from build123d import *

# Parameters (mm, degrees)
SKETCH_R     = 2
PAD_DEPTH    = 3
SKETCH001_W  = 5
SKETCH001_H  = 80
PAD001_DEPTH = 11.7
SKETCH002_R  = 1.75
SKETCH002_W  = 45
SKETCH002_H  = 10
POCKET_DEPTH = 15
SKETCH003_W  = 5
SKETCH003_H  = 80
PAD002_DEPTH = 2
FILLET_R     = 8


with BuildPart() as part:
    # Sketch → Pad (new body)
    with BuildSketch(Plane.XY):
        with BuildLine():
            Line((-14.5, 57.5), (14.5, 57.5))
            ThreePointArc((17.5, 54.5), (16.62132, 56.62132), (14.5, 57.5))
            Line((17.5, 54.5), (17.5, 45.5))
            ThreePointArc((14.5, 42.5), (16.62132, 43.37868), (17.5, 45.5))
            Line((14.5, 42.5), (5, 42.5))
            Line((5, 42.5), (5, -42.5))
            Line((5, -42.5), (14.5, -42.5))
            ThreePointArc((17.5, -45.5), (16.62132, -43.37868), (14.5, -42.5))
            Line((17.5, -45.5), (17.5, -54.5))
            ThreePointArc((14.5, -57.5), (16.62132, -56.62132), (17.5, -54.5))
            Line((14.5, -57.5), (-14.5, -57.5))
            ThreePointArc((-17.5, -54.5), (-16.62132, -56.62132), (-14.5, -57.5))
            Line((-17.5, -54.5), (-17.5, -45.5))
            ThreePointArc((-14.5, -42.5), (-16.62132, -43.37868), (-17.5, -45.5))
            Line((-5, -42.5), (-14.5, -42.5))
            Line((-5, 42.5), (-5, -42.5))
            Line((-14.5, 42.5), (-5, 42.5))
            ThreePointArc((-17.5, 45.5), (-16.62132, 43.37868), (-14.5, 42.5))
            Line((-17.5, 45.5), (-17.5, 54.5))
            ThreePointArc((-14.5, 57.5), (-16.62132, 56.62132), (-17.5, 54.5))
        make_face()
        with Locations((-10, 50)):
            Circle(SKETCH_R, mode=Mode.SUBTRACT)
        with Locations((10, 50)):
            Circle(SKETCH_R, mode=Mode.SUBTRACT)
        with Locations((-10, -50)):
            Circle(SKETCH_R, mode=Mode.SUBTRACT)
        with Locations((10, -50)):
            Circle(SKETCH_R, mode=Mode.SUBTRACT)
    extrude(amount=PAD_DEPTH)

    # Sketch001 → Pad001 (join)
    with BuildSketch(Plane.XY.offset(3)):
        with Locations((-2.5, 0)):
            Rectangle(SKETCH001_W, SKETCH001_H)
    extrude(amount=PAD001_DEPTH)

    # Sketch002 → Pocket (cut)
    with BuildSketch(Plane.YZ.offset(5)):
        with Locations((-28, 11.5)):
            Circle(SKETCH002_R)
        with Locations((28, 11.5)):
            Circle(SKETCH002_R)
        with Locations((0, 10)):
            Rectangle(SKETCH002_W, SKETCH002_H)
    extrude(amount=-POCKET_DEPTH, mode=Mode.SUBTRACT)

    # Sketch003 → Pad002 (join)
    with BuildSketch(Plane.XY.offset(3)):
        with Locations((2.5, 0)):
            Rectangle(SKETCH003_W, SKETCH003_H)
    extrude(amount=PAD002_DEPTH)

    # Fillet
    fillet_edges = [part.edges().sort_by_distance(p)[0] for p in [
        (-2.5, -40, 14.7),
        (-2.5, 40, 14.7),
    ]]
    fillet(fillet_edges, radius=FILLET_R)


solid = part.part
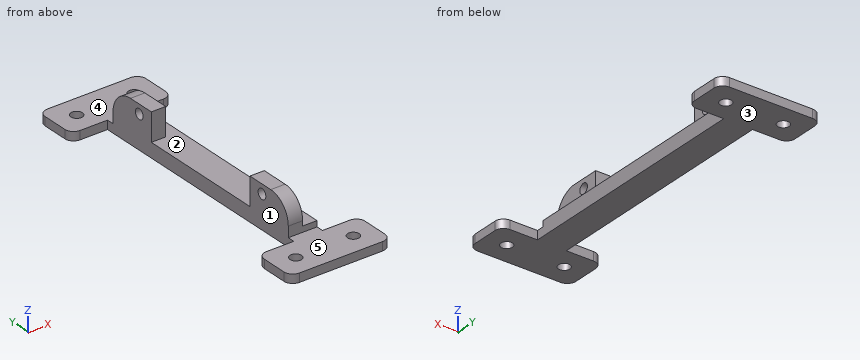
Verification items for the finished model (mm, model axes). Face numbers are marked on the shaded views. A direction names the side the tool comes from. Give positions to 0.01 mm unless a question says otherwise; leave off trailing zeros. Loops run counter-clockwise (first coordinate to the right, second up) from the corner with the lowest first, then second, coordinate; pieces in that order, holes last.
1) Sectioned sample at C-C, the plane x = -4. Enter the section's corners in (y, z), then the cut area to 3 significant figures.
2) Depth check by flat-ended pin: pin 1 Ø6 at (x, y) = (-4.5, -14) entering from +Z; pin 2 Ø5 at (y, z) = (30.5, 12) entering from +X; pin 3 Ø2.5 at (y, z) = (-12, 1.5) entering from +X; pin 4 Ø6 at (x, z) = (-5, 4.5) entering from -Y. Enter the tip coordinate at first touch or a pass-through.
3) Sectioned sample at B-B, the plane y = -28. Enter the section's corners in (x, z), then the cut area to 3 significant figures.
4) Set-up check for the marked faces 4 and 5: record each of +Z, -Z, +X, -X, +Y, -Y from which the full face is reachable in a straight line by a thin tool's end or side.
5) Sectioned sample at D-D, the plane z = 11.5. Enter the section's corners in (x, y), then the cut area to 3 significant figures.
6) Thickness scan on line 1 along Y through (x, z) = (-10, 1.15); line 2 along Y through (x, z) = (-3, 10.75); line 3 along X through (y, z) = (-25.5, 6.5). Record the ranges inside material, lowest first.
7) Sectioned sample at A-A, the plane x = 13. Enter the section's corners in (y, z).
8) Draft check along Y on the marked faces 1, 2 and 3. Enter one of: pulls with the +Y half, pulls with the -Y half, needs draft (parallel to the pull), parting line crosses it, or undercut.
Answers:
1. outline: (-57.5, 0) - (57.5, 0) - (57.5, 3) - (40, 3) - (40, 6.7) arc R8 ccw to (32, 14.7) - (22.5, 14.7) - (22.5, 5) - (-22.5, 5) - (-22.5, 14.7) - (-32, 14.7) arc R8 ccw to (-40, 6.7) - (-40, 3) - (-57.5, 3) - close; hole circle Ø3.5 at (-28, 11.5); hole circle Ø3.5 at (28, 11.5)
1. area: 798 mm2
2. pin 1: stops at z = 5
2. pin 2: stops at x = 0
2. pin 3: stops at x = 5
2. pin 4: stops at y = -57.5
3. outline: (-5, 0) - (5, 0) - (5, 5) - (0, 5) - (0, 9.75) - (-5, 9.75) - close; (-5, 13.25) - (0, 13.25) - (0, 14.7) - (-5, 14.7) - close
3. area: 81.0 mm2
4. face 4: +Z, +X, -X, +Y
4. face 5: +Z, +X, -X, -Y
5. outline: (-5, -38.4) - (0, -38.4) - (0, -29.75) - (-5, -29.75) - close; (-5, -26.25) - (0, -26.25) - (0, -22.5) - (-5, -22.5) - close; (-5, 22.5) - (0, 22.5) - (0, 26.25) - (-5, 26.25) - close; (-5, 29.75) - (0, 29.75) - (0, 38.4) - (-5, 38.4) - close
5. area: 124 mm2
6. line 1: y = -57.5 to -52, -48 to -42.5, 42.5 to 48, 52 to 57.5
6. line 2: y = -38.9 to -29.58, -26.42 to -22.5, 22.5 to 26.42, 29.58 to 38.9
6. line 3: x = -5 to 0
7. outline: (-57.5, 0) - (-42.5, 0) - (-42.5, 3) - (-57.5, 3) - close; (42.5, 0) - (57.5, 0) - (57.5, 3) - (42.5, 3) - close
8. face 1: undercut
8. face 2: undercut
8. face 3: needs draft
